```python
from build123d import *

# Parameters (mm, degrees)
F1_DEPTH = 304.8
F2_DEPTH = 304.8


with BuildPart() as f1:
    # F0 (on Front) → F1 (new body)
    with BuildSketch(Plane.XZ):
        Polygon((31.75, -6.35), (50.8, -6.35), (50.8, 6.35), (-50.8, 6.35), (-50.8, -6.35), align=None)
    extrude(amount=F1_DEPTH)

    # F0 (on Front) → F2 (join)
    with BuildSketch(Plane.XZ):
        Polygon((52.131158, -31.75), (50.8, -6.35), (31.75, -6.35), (33.081158, -31.75), align=None)
    extrude(amount=F2_DEPTH)


solid = f1.part
```
Here's how the part is built. I have some questions about the finished solid (model axes, mm). A direction names the side the tool comes from. Coordinates: 2 decimals unless noted, no trailing zeros. Order: outer loops, then holes, each group sorted by start corner. A loop starts at its lowest first (then second) coordinate and runs counter-clockwise, first axis right, second up. Notation, with made-up numbers: M -25,74 L 27,74 A16 ccw 27,96 Z; hole C -16,28.5 d11. An arc over 180 degrees is marked long. Answer as a JSON object with one key per item and string values. Group by question number.
(1) Suppose I cut it at B-B, the plane x = 21. Please give me the cut outline in (y, z), then the cut area to 3 significant figures.
(2) Which directions (+Z, -Z, +X, -X, +Y, -Y) give clear straight access to the entire face, cutting with the end or side of a thin tool? Please do faces 1 (the face through (50.8, -150, 0)), 2 (the face through (42, -150, -31.75)), 3 (the face through (-10, -150, -6.35)).
(3) I need wall thicknesses on probe 1 along Z at (x, y) = (-43, -191); probe 2 along X at (y, z) = (-265.5, 0.5); probe 3 along X at (y, z) = (-251, -25.5). Which ranges of each line are inside material? Lowest first, please.
(4) For pin 1 (6 mm diameter, centred on y = -257, z = -14.5, fed in from -X); pin 2 (1.5 mm diameter, centred on y = -200, z = -18, fed in from -X); pin 3 (6.5 mm diameter, centred on y = -90, z = -2.5, fed in from +X), each with a flat end and sliding along its axis, tell me the tip position at first contact or that it passes through.
(5) Suppose I cut it at A-A, the plane y = -201. Please give me the cut outline in (x, z), then the cut area to 3 significant figures.
(6) Suppose I cut it at C-C, the plane z = -17. Please give me the cut outline in (x, y).
Values found:
{
 "1": {"outline": "M -304.8,-6.35 L 0,-6.35 L 0,6.35 L -304.8,6.35 Z", "area": "3,870 mm^2"},
 "2": {"face 1": "+Z, +X, +Y, -Y", "face 2": "-Z, +X, -X, +Y, -Y", "face 3": "-Z, -X, +Y, -Y"},
 "3": {"probe 1": "z = -6.35 to 6.35", "probe 2": "x = -50.8 to 50.8", "probe 3": "x = 32.75 to 51.8"},
 "4": {"pin 1": "stops at x = 32.02", "pin 2": "stops at x = 32.32", "pin 3": "stops at x = 50.8"},
 "5": {"outline": "M -50.8,-6.35 L 31.75,-6.35 L 33.08,-31.75 L 52.13,-31.75 L 50.8,-6.35 L 50.8,6.35 L -50.8,6.35 Z", "area": "1,770 mm^2"},
 "6": {"outline": "M 32.31,-304.8 L 51.36,-304.8 L 51.36,0 L 32.31,0 Z"}
}
